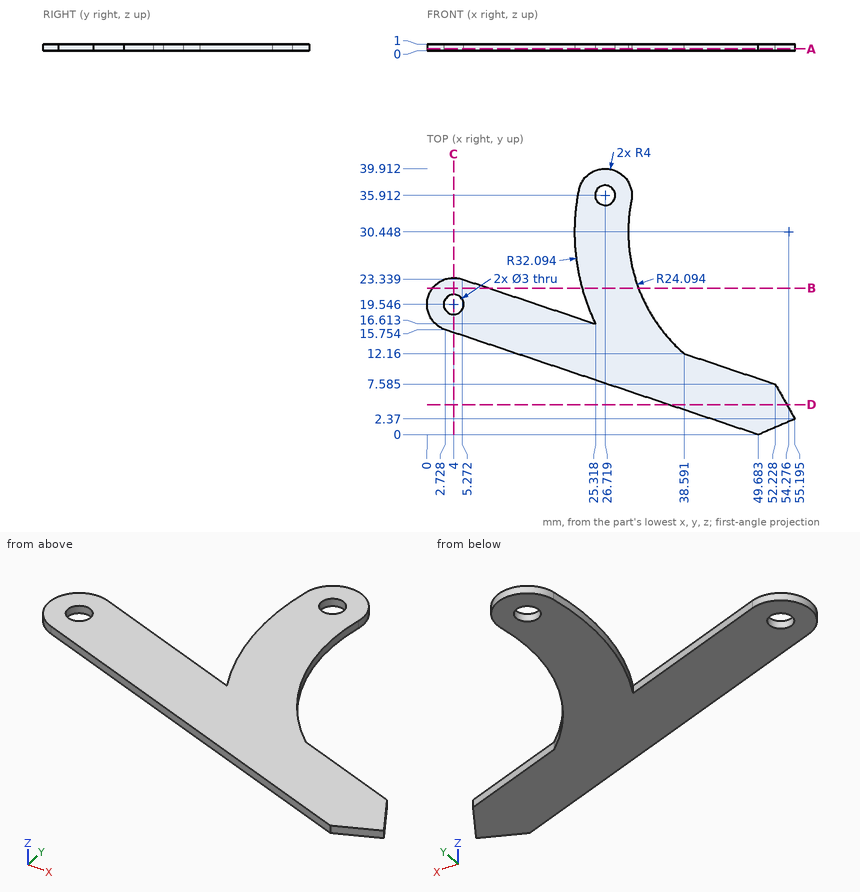
Design review of the part shown in the three views and the two pictorial views. Dimensions are in mm from the part's minimum x, y and z. Round coordinates to 2 decimals unless told otherwise and drop trailing zeros. Order: outer loops, then holes, each group sorted by start corner. A loop starts at its lowest first (then second) coordinate and runs counter-clockwise, first axis right, second up. Notation, with made-up numbers: (27.5, 47.25) -> (79.5, 47.25) arc R26 cw to (79.5, 82.25) -> close; hole circle Ø8 at (49, -7). An arc over 180 degrees is marked (long way). Write item = value, one per line. Start each with the question number.
1) Take a section at A-A on z = 0.25. State the section outline as (x, y) points (1 decimal), plus the area to 3 significant figures.
2) Take a section at C-C on x = 4. State the section outline as (y, z) points.
3) Take a section at D-D on y = 4.5. State the section outline as (x, z) points.
4) To check wall thickness, follow line 1 (Y direction, x = 4, z = 0.45) (1 decimal); line 2 (X direction, y = 31, z = 0.7); line 3 (Y direction, x = 26, z = 0.25) (1 decimal). State the ranges of each line that lie inside material, in increasing order. Write a range as from..to.
5) Take a section at B-B on y = 22. State the section outline as (x, z) points (1 decimal).
Verdict:
q1.outline = (2.7, 15.8) -> (49.7, 0) -> (55.2, 2.4) -> (52.2, 7.6) -> (38.6, 12.2) arc R24.1 cw to (30.6, 35.1) arc R4 ccw to (22.8, 36.7) arc R32.1 ccw to (25.3, 16.6) -> (5.3, 23.3) arc R4 ccw to start; hole circle Ø3 at (4, 19.5); hole circle Ø3 at (26.7, 35.9)
q1.area = 630 mm2
q2.outline = (15.33, 0) -> (18.05, 0) -> (18.05, 1) -> (15.33, 1) -> close; (21.05, 0) -> (23.55, 0) -> (23.55, 1) -> (21.05, 1) -> close
q3.outline = (36.27, 0) -> (53.98, 0) -> (53.98, 1) -> (36.27, 1) -> close
q4.line_1 = 15.3..18, 21..23.5
q4.line_2 = 22.19..30.19
q4.line_3 = 7.9..34.6, 37.2..39.8
q5.outline = (0.8, 0) -> (9.3, 0) -> (9.3, 1) -> (0.8, 1) -> close; (23.3, 0) -> (31.7, 0) -> (31.7, 1) -> (23.3, 1) -> close
